Check sheet for the modelled part. Datum: model origin and axes. Units: mm. A direction names the side the tool comes from. Round coordinates to 2 decimals unless told otherwise and drop trailing zeros. Loops run counter-clockwise (first coordinate to the right, second up) from the corner with the lowest first, then second, coordinate; pieces in that order, holes last. Notation, with made-up numbers: M -15.75,67.25 L 1.25,67.25 A22 ccw 1.25,77.25 Z; hole C 54,-27.75 d5. An arc over 180 degrees is marked long. Write item = value, one per line. Start each with the question number.
(1) Cross-section at C-C on y = -42. Record the boundary of the cut face in (x, z).
(2) Go/stop test with a flat-tipped pin: P1, Ø5, axis at x = -17.5, y = 42, coming from the -Z side. Record where the tip stops, or that it passes through.
(3) Mould release check, pull along Y, two halves, no side actions. Record for faces 3 (the face through (30, -1, 3)), 4 (the face through (0, 52, 3)), 5 (the face through (14.9, -9.5, 3)), 6 (the face through (16.075, 39.766, 3.042)): pulls with the +Y half, pulls with the -Y half, needs draft (parallel to the pull), parting line crosses it, or undercut.
(4) Set-up check for faces 1 (the face through (-15.1, 20.5, 3)), 2 (the face through (0, -52, 3)): record each of +Z, -Z, +X, -X, +Y, -Y from which the full face is reachable in a straight line by a thin tool's end or side.
(5) Scan lines: L1, parallel to X at y = 15, z = 3.2; L2, parallel to Y at x = -16.5, z = 1.65; L3, parallel to X at y = 18.5, z = 5.15. Record each from-to range of solid material in increasing order. Write a range as from..to.
(6) Cross-section at A-A on y = -13. Record the boundary of the cut face in (x, z).
(7) Cross-section at B-B on z = 2.1. State how many separate pieces and enclosed holes the cut face has, plus the area to 3 significant figures.
from build123d import *

# Parameters (mm, degrees)
SKETCH_1_W          = 60
SKETCH_1_H          = 104
EXTRUDE_1_DEPTH     = 6
CUT_EXTRUDE_1_DEPTH = 6
SKETCH_4_R          = 2.65
CUT_EXTRUDE_2_DEPTH = 6


with BuildPart() as part:
    # 草图1 → 凸台-拉伸1 (new body)
    with BuildSketch(Plane.XY):
        Rectangle(SKETCH_1_W, SKETCH_1_H)
    extrude(amount=EXTRUDE_1_DEPTH)

    # 草图2 → 切除-拉伸1 (cut)
    with BuildSketch(Plane.XY.offset(6)):
        with BuildLine():
            Line((-12.5, 18), (-12.5, 8))
            ThreePointArc((-12.5, 8), (-15, 5.5), (-17.5, 8))
            Line((-17.5, 8), (-17.5, 18))
            ThreePointArc((-17.5, 18), (-15, 20.5), (-12.5, 18))
        make_face()
        with BuildLine():
            Line((17.5, 18), (17.5, 8))
            ThreePointArc((17.5, 8), (15, 5.5), (12.5, 8))
            Line((12.5, 8), (12.5, 18))
            ThreePointArc((12.5, 18), (15, 20.5), (17.5, 18))
        make_face()
        with BuildLine():
            Line((17.5, -12), (17.5, -22))
            ThreePointArc((17.5, -22), (15, -24.5), (12.5, -22))
            Line((12.5, -22), (12.5, -12))
            ThreePointArc((12.5, -12), (15, -9.5), (17.5, -12))
        make_face()
        with BuildLine():
            Line((-12.5, -12), (-12.5, -22))
            ThreePointArc((-12.5, -22), (-15, -24.5), (-17.5, -22))
            Line((-17.5, -22), (-17.5, -12))
            ThreePointArc((-17.5, -12), (-15, -9.5), (-12.5, -12))
        make_face()
    extrude(amount=-CUT_EXTRUDE_1_DEPTH, mode=Mode.SUBTRACT)

    # 草图4 → 切除-拉伸2 (cut)
    with BuildSketch(Plane.XY.offset(6)):
        with Locations((-17.5, 42)):
            Circle(SKETCH_4_R)
        with Locations((-17.5, -42)):
            Circle(SKETCH_4_R)
        with Locations(Location((17.5, -42, 0), (0, 0, 180))):
            Circle(SKETCH_4_R)
        with Locations(Location((17.5, 42, 0), (0, 0, 180))):
            Circle(SKETCH_4_R)
    extrude(amount=-CUT_EXTRUDE_2_DEPTH, mode=Mode.SUBTRACT)


solid = part.part
Result:
q1.outline = M -30,0 L -20.15,0 L -20.15,6 L -30,6 Z; M -14.85,0 L 14.85,0 L 14.85,6 L -14.85,6 Z; M 20.15,0 L 30,0 L 30,6 L 20.15,6 Z
q2.P1 = through
q3.face_3 = needs draft
q3.face_4 = pulls with the +Y half
q3.face_5 = undercut
q3.face_6 = undercut
q4.face_1 = +Z, -Z
q4.face_2 = +Z, -Z, +X, -X, -Y
q5.L1 = -30..-17.5, -12.5..12.5, 17.5..30
q5.L2 = -52..-44.45, -39.55..-24, -10..6, 20..39.55, 44.45..52
q5.L3 = -30..-17.45, -12.55..12.55, 17.45..30
q6.outline = M -30,0 L -17.5,0 L -17.5,6 L -30,6 Z; M -12.5,0 L 12.5,0 L 12.5,6 L -12.5,6 Z; M 17.5,0 L 30,0 L 30,6 L 17.5,6 Z
q7.separate_pieces = 1
q7.enclosed_holes = 8
q7.area = 5,870 mm^2
